from build123d import *

# Parameters (mm, degrees)
BO_ALTMA1_T           = -1.5
MENFEZ1_START         = -35.355339059
MENFEZ1_DEPTH         = 1.5
IZIM6_R               = 2.5
KES_EKSTR_ZYON2_DEPTH = 111.566722087
KES_EKSTR_ZYON3_DEPTH = 10
IZIM9_R               = 1.5
KES_EKSTR_ZYON4_DEPTH = 0.1
KUBBE2_FACE_RADIUS    = 1.5
KUBBE2_HEIGHT         = 1.3
KES_EKSTR_ZYON5_START = -0.1
IZIM10_R              = 1.5
KES_EKSTR_ZYON5_DEPTH = 0.1
KUBBE3_FACE_RADIUS    = 1.5
KUBBE3_HEIGHT         = 1.3
KES_EKSTR_ZYON6_REACH = 112.567
IZIM11_R              = 1.25


# Read off the part's stored shape, not the designer's step: Menfez1
with BuildPart() as part:
    # Çizim2 → Loft1 section 0
    with BuildSketch(Plane.XY.offset(40)):
        with BuildLine():
            Line((-25, 50), (25, 50))
            Line((25, 50), (25, -10))
            Line((25, -10), (-25, -10))
            Line((-25, -10), (-25, 50))
        make_face()
    # Çizim1 → Loft1 section 1
    with BuildSketch(Plane.XY):
        with BuildLine():
            Line((-25, 50), (25, 50))
            Line((25, 50), (25, -50))
            Line((25, -50), (-25, -50))
            Line((-25, -50), (-25, 50))
        make_face()
    loft()

    # İç Boşaltma1
    bo_altma1_openings = [part.faces().sort_by_distance(p)[0] for p in [
        (0, 0, 0),
    ]]
    offset(amount=BO_ALTMA1_T, openings=bo_altma1_openings, kind=Kind.INTERSECTION)

    # Menfez1 outline → Menfez1 (cut)
    with BuildSketch(Plane(origin=(0, 0, 0), x_dir=(1, 0, 0), z_dir=(0, 0.707106781186547, -0.7071067811865479)).offset(MENFEZ1_START)):
        with BuildLine():
            add(Edge.make_bspline(
                [(22.5, 7.071067812), (22.5, 5.598458472), (22.209921279, 2.653239791), (20.921288378, -1.594813577), (18.828662098, -5.509841982), (16.012460892, -8.94139308), (12.580909794, -11.757594286), (8.665881389, -13.850220566), (4.417828021, -15.138853467), (0, -15.573971549), (-4.417828021, -15.138853467), (-8.665881389, -13.850220566), (-12.580909794, -11.757594286), (-16.012460892, -8.94139308), (-18.828662098, -5.509841982), (-20.921288378, -1.594813577), (-22.209921279, 2.653239791), (-22.645039361, 7.071067812), (-22.209921279, 11.488895833), (-20.921288378, 15.7369492), (-18.828662098, 19.651977606), (-16.012460892, 23.083528704), (-12.580909794, 25.89972991), (-8.665881389, 27.99235619), (-4.417828021, 29.280989091), (0, 29.716107172), (4.417828021, 29.280989091), (8.665881389, 27.99235619), (12.580909794, 25.89972991), (16.012460892, 23.083528704), (18.828662098, 19.651977606), (20.921288378, 15.7369492), (22.209921279, 11.488895833), (22.5, 8.543677152), (22.5, 7.071067812)],
                knots=[0, 0, 0, 0, 0.03125, 0.0625, 0.09375, 0.125, 0.15625, 0.1875, 0.21875, 0.25, 0.28125, 0.3125, 0.34375, 0.375, 0.40625, 0.4375, 0.46875, 0.5, 0.53125, 0.5625, 0.59375, 0.625, 0.65625, 0.6875, 0.71875, 0.75, 0.78125, 0.8125, 0.84375, 0.875, 0.90625, 0.9375, 0.96875, 1, 1, 1, 1], degree=3))
        make_face()
    extrude(amount=MENFEZ1_DEPTH, mode=Mode.SUBTRACT)

    # Çizim6 → Kes-Ekstrüzyon2 (cut, through all)
    with BuildSketch(Plane(origin=(0, 50, 0), x_dir=(1, 0, 0), z_dir=(0, 1, 0))):
        with Locations(Location((0, -20, 0), (0, 0, 270))):
            Circle(IZIM6_R)
    extrude(amount=-KES_EKSTR_ZYON2_DEPTH, mode=Mode.SUBTRACT)

    # Çizim7 → Kes-Ekstrüzyon3 (cut)
    with BuildSketch(Plane(origin=(0, -50, 0), x_dir=(1, 0, 0), z_dir=(0, 1, 0))):
        Polygon((19.573356646, -1), (20.223356646, -2.125833025), (18.923356646, -2.125833025), align=None)
        Polygon((-0.426643354, -1), (0.223356646, -2.125833025), (-1.076643354, -2.125833025), align=None)
        Polygon((-20.426643354, -1), (-19.776643354, -2.125833025), (-21.076643354, -2.125833025), align=None)
    extrude(amount=KES_EKSTR_ZYON3_DEPTH, mode=Mode.SUBTRACT)

    # Çizim9 → Kes-Ekstrüzyon4 (cut)
    with BuildSketch(Plane(origin=(-23.5, 0, 0), x_dir=(0, 0, -1), z_dir=(1, 0, 0))):
        with Locations(Location((-6, -23.5, 0), (0, 0, 90))):
            Circle(IZIM9_R)
    extrude(amount=-KES_EKSTR_ZYON4_DEPTH, mode=Mode.SUBTRACT)

    # Kubbe2: a dome of height H over a round flat face of radius A is a cap of a sphere of radius (A * A + H * H) / (2 * H)
    kubbe2_r = (KUBBE2_FACE_RADIUS * KUBBE2_FACE_RADIUS + KUBBE2_HEIGHT * KUBBE2_HEIGHT) / (2 * KUBBE2_HEIGHT)
    kubbe2_base = Plane((-23.6, -23.5, 6), z_dir=(-1, 0, 0))
    with Locations(kubbe2_base.offset(KUBBE2_HEIGHT - kubbe2_r)):
        kubbe2_ball = Sphere(kubbe2_r, mode=Mode.PRIVATE)
    add(split(kubbe2_ball, bisect_by=kubbe2_base, keep=Keep.TOP, mode=Mode.PRIVATE), mode=Mode.SUBTRACT)

    # Çizim10 → Kes-Ekstrüzyon5 (cut)
    with BuildSketch(Plane.ZY.offset(-23.5).offset(KES_EKSTR_ZYON5_START)):
        with Locations(Location((6, -23.5, 0), (0, 0, 90))):
            Circle(IZIM10_R)
    extrude(amount=KES_EKSTR_ZYON5_DEPTH, mode=Mode.SUBTRACT)

    # Kubbe3: a dome of height H over a round flat face of radius A is a cap of a sphere of radius (A * A + H * H) / (2 * H)
    kubbe3_r = (KUBBE3_FACE_RADIUS * KUBBE3_FACE_RADIUS + KUBBE3_HEIGHT * KUBBE3_HEIGHT) / (2 * KUBBE3_HEIGHT)
    kubbe3_base = Plane((23.6, -23.5, 6), z_dir=(1, 0, 0))
    with Locations(kubbe3_base.offset(KUBBE3_HEIGHT - kubbe3_r)):
        kubbe3_ball = Sphere(kubbe3_r, mode=Mode.PRIVATE)
    add(split(kubbe3_ball, bisect_by=kubbe3_base, keep=Keep.TOP, mode=Mode.PRIVATE), mode=Mode.SUBTRACT)

    # Çizim11 → Kes-Ekstrüzyon6 (cut, up to next)
    with BuildSketch(Plane(origin=(0, 50, 0), x_dir=(1, 0, 0), z_dir=(0, 1, 0)), mode=Mode.PRIVATE) as kes_ekstr_zyon6_sk1:
        with Locations(Location((21.5, -6, 0), (0, 0, 270))):
            Circle(IZIM11_R)
    kes_ekstr_zyon6_tool1 = extrude(kes_ekstr_zyon6_sk1.sketch, amount=-KES_EKSTR_ZYON6_REACH, mode=Mode.PRIVATE) & part.part
    # Çizim11 → Kes-Ekstrüzyon6 (cut, up to next)
    with BuildSketch(Plane(origin=(0, 50, 0), x_dir=(1, 0, 0), z_dir=(0, 1, 0)), mode=Mode.PRIVATE) as kes_ekstr_zyon6_sk2:
        with Locations(Location((-21.5, -6, 0), (0, 0, 270))):
            Circle(IZIM11_R)
    kes_ekstr_zyon6_tool2 = extrude(kes_ekstr_zyon6_sk2.sketch, amount=-KES_EKSTR_ZYON6_REACH, mode=Mode.PRIVATE) & part.part
    add(kes_ekstr_zyon6_tool1.solids().sort_by_distance((21.5, 50, 6))[0], mode=Mode.SUBTRACT)
    add(kes_ekstr_zyon6_tool2.solids().sort_by_distance((-21.5, 50, 6))[0], mode=Mode.SUBTRACT)


solid = part.part
Check sheet for the modelled part. Datum: model origin and axes. Units: mm. A direction names the side the tool comes from. Give positions to 0.01 mm unless a question says otherwise; leave off trailing zeros. Answer as CSV lines item,"result". Start each with the question number.
Item 1: Gauge pin test, flat ends, axial feed: P1, Ø12, axis at x = -1, z = 22, coming from the -Y side; P2, Ø1.4, axis at x = -20.5, y = -47, coming from the -Z side; P3, Ø3, axis at x = -17, z = 10, coming from the -Y side. Record the tip position at first contact, or that the pin passes through.
Item 2: Thickness scan on line 1 (X direction, y = 49.55, z = 6); line 2 (X direction, y = 40, z = 18); line 3 (Z direction, x = 11.5, y = 27). Record the ranges inside material, lowest first. Write a range as [from, to].
Item 3: Mould release check, pull along Y, two halves, no side actions. Record for faces 1 (the face through (0.1, 49.3, 17.5)), 2 (the face through (23, -30, 20)), 3 (the face through (-23.5, 11, 18)): +Y half, -Y half, draft (parallel to the pull), parting line (faces both ways), or undercut.
Item 4: Cross-section at A-A on z = 6. State how many separate pieces and enclosed holes the cut face has, plus the area to 3 significant figures.
Item 5: Tool access check on faces 4 (the face through (0, 21, 40)), 5 (the face through (23.5, 13, 18)), 6 (the face through (20.28, 49.26, 5.73)). Record the directions out of +Z, -Z, +X, -X, +Y, -Y that give a thin tool (end or side, any length) a straight path to the whole face; none if there is none.
Established:
1,P1,"stops at y = 48.5"
1,P2,"stops at z = 0.18"
1,P3,"stops at y = -41.5"
2,line 1,"x = [-25, -22.75], [-20.25, 20.25], [22.75, 25]"
2,line 2,"x = [-25, -23.5], [23.5, 25]"
2,line 3,"z = [38.5, 40]"
3,face 1,"draft"
3,face 2,"-Y half"
3,face 3,"undercut"
4,separate pieces,"3"
4,enclosed holes,"0"
4,area,"388 mm^2"
5,face 4,"+Z, +X, -X, +Y, -Y"
5,face 5,"-Z"
5,face 6,"+Y"
